Source: CAD feature listing. Evaluate the final solid. Frame: model axes, mm. A direction names the side the tool comes from. Round coordinates to 2 decimals unless told otherwise and drop trailing zeros. Order: outer loops, then holes, each group sorted by start corner. A loop starts at its lowest first (then second) coordinate and runs counter-clockwise, first axis right, second up.
```python
from build123d import *

# Parameters (mm, degrees)
F0_W     = 247.035488
F0_H     = 56.043873
F1_DEPTH = 32.512
F2_R     = 11.307097
F3_DEPTH = 43.434
F4_W     = 143.55097
F4_H     = 56.043873
F5_DEPTH = 45.212


with BuildPart() as f1:
    # F0 (on Top) → F1 (new body)
    with BuildSketch(Plane.XY):
        with Locations((0, 1.966451)):
            Rectangle(F0_W, F0_H)
    extrude(amount=F1_DEPTH)

    # F2 (on face) → F3 (cut)
    with BuildSketch(Plane.XY.offset(32.512)):
        with Locations((100.411944, 0)):
            Circle(F2_R)
        with Locations((-97.708069, 0)):
            Circle(F2_R)
    extrude(amount=-F3_DEPTH, mode=Mode.SUBTRACT)

    # F4 (on face) → F5 (join)
    with BuildSketch(Plane.XY.offset(32.512)):
        with Locations((2.089355, 1.966451)):
            Rectangle(F4_W, F4_H)
    extrude(amount=F5_DEPTH)


solid = f1.part
```
1. Access query for faces 5 (the face through (-109, 2, 32.512)), 6 (the face through (-2, 2, 0)), 7 (the face through (93, 9, 32.512)). Directions: +Z, -Z, +X, -X, +Y, -Y. A direction counts if a zero-diameter tool reaches every point of the face in a straight line with its end or side. Return the directions, or none.
2. Pull-direction query (X, two-part tool) for faces 1 (the face through (-123.518, 2, 16)), 2 (the face through (-2, 29.988, 30)), 3 (the face through (123.518, 2, 16)), 4 (the face through (111.197, 3.396, 16.484)); classes: released by +X, released by -X, zero draft, split by the parting line, or undercut.
3. Section C-C on z = 19.5. Return loops of the section in (x, y).
4. Section D-D on y = -18. Return loops of the section in (x, z).
5. Section B-B on x = 97. Return loops of the section in (y, z).
6. First-contact query: pin 1 (4 mm diameter, centred on x = 7, y = -15, fed in from -Z); pin 2 (25 mm diameter, centred on x = 105, y = 12, fed in from +Z); pin 3 (22.5 mm diameter, centred on y = -6, z = 52.5, fed in from +X); pin 4 (13.5 mm diameter, centred on y = 9, z = 58.5, fed in from -X). Flat tips, straight axial feed; report the tip coordinate or a pass-through.
7. Section A-A on y = 0. Return loops of the section in (x, z), plus the area to 3 significant figures.
8. Line query: line 1 along X through (y, z) = (3.5, 18); line 2 along Z through (x, y) = (92.5, 21); line 3 along X through (y, z) = (10, 40.5). Output: solid intervals per line, ascending.
Result:
1. face 5: +Z, -X, +Y, -Y
1. face 6: -Z, +X, -X, +Y, -Y
1. face 7: +Z, +X, +Y, -Y
2. face 1: released by -X
2. face 2: zero draft
2. face 3: released by +X
2. face 4: undercut
3. outline: (-123.52, -26.06) - (123.52, -26.06) - (123.52, 29.99) - (-123.52, 29.99) - close; hole circle Ø22.61 at (-97.71, 0); hole circle Ø22.61 at (100.41, 0)
4. outline: (-123.52, 0) - (123.52, 0) - (123.52, 32.51) - (73.86, 32.51) - (73.86, 77.72) - (-69.69, 77.72) - (-69.69, 32.51) - (-123.52, 32.51) - close
5. outline: (-26.06, 0) - (-10.78, 0) - (-10.78, 32.51) - (-26.06, 32.51) - close; (10.78, 0) - (29.99, 0) - (29.99, 32.51) - (10.78, 32.51) - close
6. pin 1: stops at z = 0
6. pin 2: stops at z = 32.51
6. pin 3: stops at x = 73.86
6. pin 4: stops at x = -69.69
7. outline: (-123.52, 0) - (-109.02, 0) - (-109.02, 32.51) - (-123.52, 32.51) - close; (-86.4, 0) - (89.1, 0) - (89.1, 32.51) - (73.86, 32.51) - (73.86, 77.72) - (-69.69, 77.72) - (-69.69, 32.51) - (-86.4, 32.51) - close; (111.72, 0) - (123.52, 0) - (123.52, 32.51) - (111.72, 32.51) - close
7. area: 13,100 mm2
8. line 1: x = -123.52 to -108.46, -86.96 to 89.66, 111.16 to 123.52
8. line 2: z = 0 to 32.51
8. line 3: x = -69.69 to 73.86
